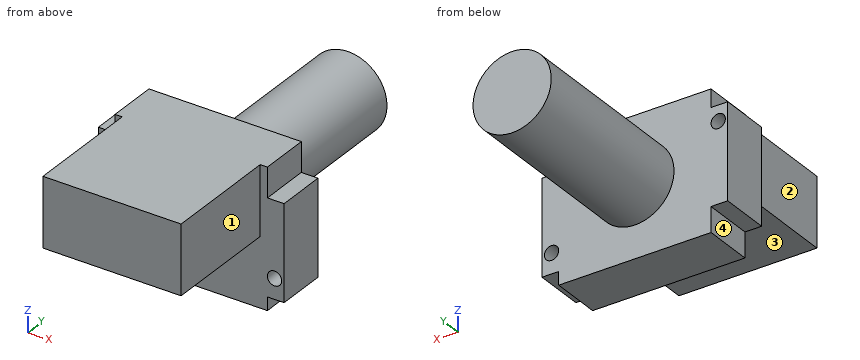
from build123d import *

# Parameters (mm, degrees)
SKETCH_1_W          = 29
SKETCH_1_H          = 14.5
EXTRUDE_1_DEPTH     = 24.5
SKETCH_3_W          = 32
SKETCH_3_H          = 29
EXTRUDE_3_DEPTH     = 10.5
SKETCH_6_W          = 20
SKETCH_6_H          = 10.5
EXTRUDE_5_DEPTH     = 3.5
SKETCH_8_W          = 20
SKETCH_8_H          = 10.5
EXTRUDE_6_DEPTH     = 3.5
SKETCH_9_R          = 1.5
CUT_EXTRUDE_1_DEPTH = 36
SKETCH_11_R         = 8.217115379
EXTRUDE_7_DEPTH     = 38


with BuildPart() as part:
    # 草圖1 → 填料-伸長1 (new body)
    with BuildSketch(Plane(origin=(0, 0, 0), x_dir=(1, 0, 0), z_dir=(0, 1, 0))):
        Rectangle(SKETCH_1_W, SKETCH_1_H)
    extrude(amount=EXTRUDE_1_DEPTH)

    # 草圖3 → 填料-伸長3 (add)
    with BuildSketch(Plane(origin=(0, 24.5, 0), x_dir=(1, 0, 0), z_dir=(0, 1, 0))):
        with Locations((0, 7.25)):
            Rectangle(SKETCH_3_W, SKETCH_3_H)
    extrude(amount=EXTRUDE_3_DEPTH)

    # 草圖6 → 填料-伸長5 (add)
    with BuildSketch(Plane(origin=(16, 0, 0), x_dir=(0, 0, -1), z_dir=(1, 0, 0))):
        with Locations((8.978907639, 29.75)):
            Rectangle(SKETCH_6_W, SKETCH_6_H)
    extrude(amount=EXTRUDE_5_DEPTH)

    # 草圖8 → 填料-伸長6 (add)
    with BuildSketch(Plane.ZY.offset(16)):
        with Locations((-6.503080988, 29.75)):
            Rectangle(SKETCH_8_W, SKETCH_8_H)
    extrude(amount=EXTRUDE_6_DEPTH)

    # 草圖9 → 除料-伸長1 (cut, through all)
    with BuildSketch(Plane(origin=(0, 35, 0), x_dir=(1, 0, 0), z_dir=(0, 1, 0))):
        with Locations((17.5, 14.75)):
            Circle(SKETCH_9_R)
        with Locations((-17.5, -0.25)):
            Circle(SKETCH_9_R)
    extrude(amount=-CUT_EXTRUDE_1_DEPTH, mode=Mode.SUBTRACT)

    # 草圖11 → 填料-伸長7 (add)
    with BuildSketch(Plane(origin=(0, 35, 0), x_dir=(1, 0, 0), z_dir=(0, 1, 0))):
        with Locations((0, 6.709500823)):
            Circle(SKETCH_11_R)
    extrude(amount=EXTRUDE_7_DEPTH)


solid = part.part
CAD build for the part. Positions are in the model's coordinates, mm. Face numbers are marked on the shaded views. A direction names the side the tool comes from. Give positions to 0.01 mm unless a question says otherwise; leave off trailing zeros. Order: outer loops, then holes, each group sorted by start corner. A loop starts at its lowest first (then second) coordinate and runs counter-clockwise, first axis right, second up. Notation, with made-up numbers: (35, 54) - (81, 54) arc R23 cw to (81, 77) - close; hole circle Ø10 at (-37, -17). An arc over 180 degrees is marked (long way). Answer in a Markdown table with one row per item.
1. Probe probe 1 along X at (y, z) = (32, 0.25); probe 2 along Z at (x, y) = (-6, 6.5); probe 3 along Y at (x, z) = (16, -7). List the from-to ranges inside material, lowest first. Write a range as [from, to].
Data:
| item | result |
|---|---|
| probe 1 | x = [-19.5, -19], [-16, 19.5] |
| probe 2 | z = [-7.25, 7.25] |
| probe 3 | y = [24.5, 35] |
2. Saw through at A-A, the plane x = -17.5. Give the cut face in (y, z), plus the area to 4 significant figures.
Data:
| item | result |
|---|---|
| outline | (24.5, -16.5) - (35, -16.5) - (35, -1.25) - (24.5, -1.25) - close; (24.5, 1.75) - (35, 1.75) - (35, 3.5) - (24.5, 3.5) - close |
| area | 178.5 mm² |
3. Saw through at B-B, the plane z = 0.25. Give the cut face in (x, y), plus the area to 3 significant figures.
Data:
| item | result |
|---|---|
| outline | (-19.5, 24.5) - (-19, 24.5) - (-19, 35) - (-19.5, 35) - close; (-16, 24.5) - (-14.5, 24.5) - (-14.5, 0) - (14.5, 0) - (14.5, 24.5) - (19.5, 24.5) - (19.5, 35) - (4.37, 35) - (4.37, 73) - (-4.37, 73) - (-4.37, 35) - (-16, 35) - close |
| area | 1,420 mm² |
4. Tool access for the marked faces 1, 2, 3 and 4: list every direction of +Z, -Z, +X, -X, +Y, -Y with a clear straight run to the whole face (end or side of a thin tool).
Data:
| item | result |
|---|---|
| face 1 | +Z, -Z, +X, -Y |
| face 2 | +Z, -Z, -X, -Y |
| face 3 | -Z, +X, -X, -Y |
| face 4 | -Z, -X, +Y, -Y |
5. Saw through at C-C, the plane x = 12. Give the cut face in (y, z), plus the area to 3 significant figures.
Data:
| item | result |
|---|---|
| outline | (0, -7.25) - (24.5, -7.25) - (24.5, -21.75) - (35, -21.75) - (35, 7.25) - (0, 7.25) - close |
| area | 660 mm² |
6. Flat gauge pins, fed straight in: pin 1 (1.1 mm diameter, centred on y = 31.5, z = 5, fed in from -X); pin 2 (2.5 mm diameter, centred on x = -17.5, z = 0.25, fed in from +Y); pin 3 (1 mm diameter, centred on y = 59, z = -9.5, fed in from +X); pin 4 (11.5 mm diameter, centred on y = 12, z = 0, fed in from +X). Where does each tip first touch, or does it go through?
Data:
| item | result |
|---|---|
| pin 1 | stops at x = -16 |
| pin 2 | passes through |
| pin 3 | stops at x = 7.89 |
| pin 4 | stops at x = 14.5 |
7. Saw through at D-D, the plane y = 7. Give the cut face in (x, z).
Data:
| item | result |
|---|---|
| outline | (-14.5, -7.25) - (14.5, -7.25) - (14.5, 7.25) - (-14.5, 7.25) - close |
